```python
from build123d import *

# Parameters (mm, degrees)
F0_W          = 20.5
F0_H          = 12
F1_DEPTH      = 5.5
F1_DEPTH_BACK = 5.5
F2_R          = 2
F3_DEPTH      = 4.5
F4_R          = 2
F5_DEPTH      = 7.5
F6_W          = 1
F6_H          = 5
F7_DEPTH      = 2


with BuildPart() as f1:
    # F0 (on Top) → F1 (new body, two sides)
    with BuildSketch(Plane.XY) as f1_sk:
        Rectangle(F0_W, F0_H)
    extrude(amount=F1_DEPTH)
    extrude(f1_sk.sketch, amount=-F1_DEPTH_BACK)

    # F2 (on face) → F3 (join)
    with BuildSketch(Plane(origin=(-10.25, 0, 0), x_dir=(0, -1, 0), z_dir=(-1, 0, 0))):
        Circle(F2_R)
    extrude(amount=F3_DEPTH)

    # F4 (on face) → F5 (join)
    with BuildSketch(Plane.YZ.offset(10.25)):
        Circle(F4_R)
    extrude(amount=F5_DEPTH)

    # F6 (on face) → F7 (join)
    with BuildSketch(Plane(origin=(0, 0, -5.5), x_dir=(1, 0, 0), z_dir=(0, 0, -1))):
        with Locations((-8.75, 0)):
            Rectangle(F6_W, F6_H)
    extrude(amount=F7_DEPTH)


solid = f1.part
```
Geometry: final body of the model. Coordinates: model frame, mm. A direction names the side the tool comes from. Coordinates: 2 decimals unless noted, no trailing zeros. Order: outer loops, then holes, each group sorted by start corner. A loop starts at its lowest first (then second) coordinate and runs counter-clockwise, first axis right, second up. Notation, with made-up numbers: (38.25, 24.5) -> (76.25, 24.5) arc R10 ccw to (76.25, 39.5) -> close; hole circle Ø6 at (17.25, 67). An arc over 180 degrees is marked (long way). Use CSV: the item, a comma, the result in double quotes.
1) Section C-C on x = 5. Output: boundary loops of the cut face in (y, z), then the cut area to 3 significant figures.
Findings:
outline,"(-6, -5.5) -> (6, -5.5) -> (6, 5.5) -> (-6, 5.5) -> close"
area,"132 mm^2"
2) Section D-D on z = -6.25. Output: boundary loops of the cut face in (x, y).
Findings:
outline,"(-9.25, -2.5) -> (-8.25, -2.5) -> (-8.25, 2.5) -> (-9.25, 2.5) -> close"
3) Pin query (flat end, axial travel): pin 1 Ø2 at (x, z) = (12, 1.5) entering from -Y; pin 2 Ø2 at (y, z) = (-1, -4) entering from +X; pin 3 Ø3 at (x, z) = (14.5, 2.5) entering from +Y. Return the tip coordinate at first contact, or that it passes through.
Findings:
pin 1,"stops at y = -1.94"
pin 2,"stops at x = 10.25"
pin 3,"stops at y = 1.73"
4) Section B-B on y = 0. Output: boundary loops of the cut face in (x, z).
Findings:
outline,"(-14.75, -2) -> (-10.25, -2) -> (-10.25, -5.5) -> (-9.25, -5.5) -> (-9.25, -7.5) -> (-8.25, -7.5) -> (-8.25, -5.5) -> (10.25, -5.5) -> (10.25, -2) -> (17.75, -2) -> (17.75, 2) -> (10.25, 2) -> (10.25, 5.5) -> (-10.25, 5.5) -> (-10.25, 2) -> (-14.75, 2) -> close"
5) Access query for faces 1 (the flat face through (-10.25, 0, 3)), 2 (the cylindrical face through (14, 0, -2)), 3 (the flat face through (-9, 2.5, -6)). Directions: +Z, -Z, +X, -X, +Y, -Y. A direction counts if a zero-diameter tool reaches every point of the face in a straight line with its end or side. Return the directions, or none.
Findings:
face 1,"-X"
face 2,"+X"
face 3,"-Z, +X, -X, +Y"
6) Line query: line 1 (Z direction, x = 3.5, y = 3.5); line 2 (X direction, y = -5, z = 4.75); line 3 (X direction, y = 1.25, z = -5.75). Output: solid intervals per line, ascending.
Findings:
line 1,"z = -5.5 to 5.5"
line 2,"x = -10.25 to 10.25"
line 3,"x = -9.25 to -8.25"
7) Section A-A on z = 0. Output: boundary loops of the cut face in (x, y), then the cut area to 3 significant figures.
Findings:
outline,"(-14.75, -2) -> (-10.25, -2) -> (-10.25, -6) -> (10.25, -6) -> (10.25, -2) -> (17.75, -2) -> (17.75, 2) -> (10.25, 2) -> (10.25, 6) -> (-10.25, 6) -> (-10.25, 2) -> (-14.75, 2) -> close"
area,"294 mm^2"
